from build123d import *


with BuildPart() as part:
    # Sketch1 → Revolve1 (revolve)
    with BuildSketch(Plane(origin=(0, 0, 0), x_dir=(1, 0, 0), z_dir=(0, 1, 0))):
        Polygon((0, 44.45), (0, 0), (63.5, 0), (63.5, 3.175), (60.325, 3.175), (60.325, 7.9375), (63.5, 7.9375), (63.5, 11.1125), (60.325, 11.1125), (60.325, 15.875), (63.5, 15.875), (63.5, 19.05), (50.8, 19.05), (50.8, 38.1), (63.5, 38.1), (63.5, 50.8), (79.375, 50.8), (79.375, 31.75), (92.075, 31.75), (92.075, 76.2), (12.7, 76.2), (12.7, 63.5), (38.1, 63.5), (38.1, 44.45), align=None)
    revolve(axis=Axis((0, 0, -44.45), (0, 0, 1)))


solid = part.part
Input: part model. Units: mm. Frame: model coordinates. A direction names the side the tool comes from. Round coordinates to 2 decimals unless told otherwise and drop trailing zeros.
1) Reachability of faces 5 (the flat face through (-1, -19, -76.2)), 6 (the flat face through (-16, 1, -63.5)), 7 (the cylindrical face through (-13.77, -61.99, -44.54)) from +Z, -Z, +X, -X, +Y, -Y: full face, straight path, thin tool, end or side. Return the list, or none.
2) Ray query, L1, parallel to Y at x = 0, z = -37 (3 decimals); L2, parallel to Z at x = 13, y = 16; L3, parallel to Y at x = 0, z = -57.5 (3 decimals). Return the intervals inside material, ascending.
3) Draft query along Z for faces 1 (the flat face through (-40, 69, -31.75)), 2 (the flat face through (-56, -23, -15.875)), 3 (the flat face through (-29, 43, -19.05)), 4 (the cylindrical face through (-2.75, -12.4, -69.76)). Return one class per face: pulls with the +Z half, pulls with the -Z half, needs draft (parallel to the pull), parting line crosses it, or undercut.
4) Contact query for flat-ended pins moving along their axis: P1, Ø3, axis at x = 31.5, z = -26, coming from the +Y side; P2, Ø3, axis at x = -53.5, z = -12, coming from the -Y side; P3, Ø12, axis at y = -14.5, z = -17, coming from the -X side. Output: stop coordinate, or through.
Geometry says:
1. face 5: -Z, +X, -X, +Y, -Y
1. face 6: none
1. face 7: +Z
2. L1: y = -92.075 to -79.375, -50.8 to 50.8, 79.375 to 92.075
2. L2: z = -76.2 to -63.5, -44.45 to 0
2. L3: y = -92.075 to -38.1, 38.1 to 92.075
3. face 1: pulls with the +Z half
3. face 2: undercut
3. face 3: undercut
3. face 4: needs draft
4. P1: stops at y = 41
4. P2: stops at y = -36.03
4. P3: stops at x = -62.93
